The drawing under review shows one solid part. Ordinate dimensions are in mm from its lowest x, y, z. Give positions to 0.01 mm unless a question says otherwise; leave off trailing zeros. Loops run counter-clockwise (first coordinate to the right, second up) from the corner with the lowest first, then second, coordinate; pieces in that order, holes last. Notation, with made-up numbers: M 48,50 L 97,50 A13 cw 97,73 Z; hole C -35,24 d1. An arc over 180 degrees is marked long. One line per item, written item: value. Start each with the question number.
Q1. We need section C-C on y = 0.5. Write out the cut boundary in (x, z), plus the area to 3 significant figures.
Q2. For pin 1 (1.5 mm diameter, centred on y = 1, z = 1.5, fed in from -X), flat-tipped, find the tip position at first contact; note if it passes through.
Q3. We need section B-B on z = 2.4. Write out the cut boundary in (x, y).
Q4. We need section A-A on x = 19. Write out the cut boundary in (y, z), plus the area to 3 significant figures.
Q5. To check wall thickness, follow line 1 along Y through (x, z) = (6, 2.05); line 2 along Z through (x, y) = (20, 1.05); line 3 along Z through (x, y) = (12, 0.25). State the ranges of each line that lie inside material, in increasing order. Write a range as from..to.
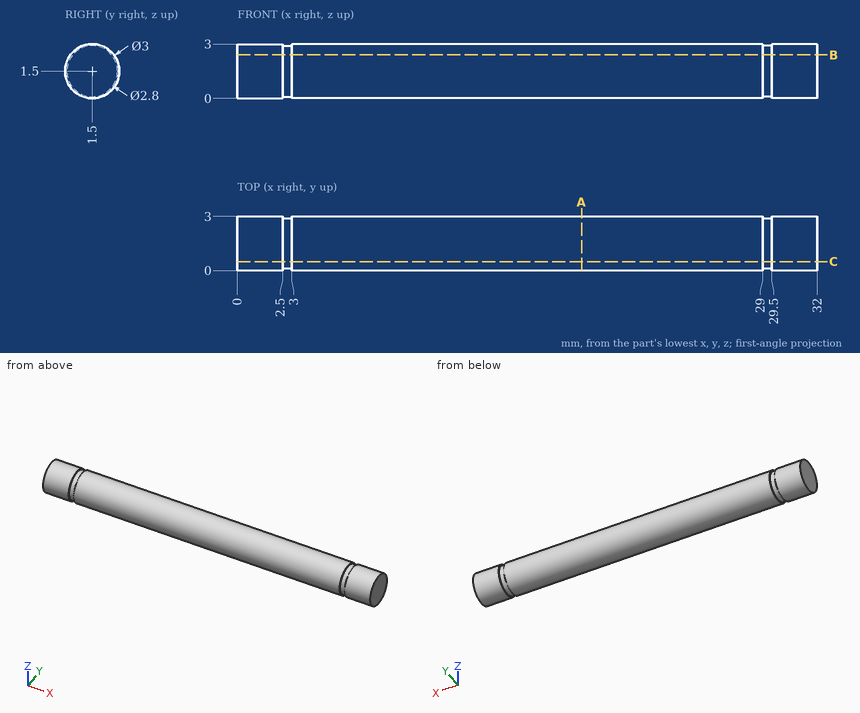
Solved:
1. outline: M 0,0.38 L 2.5,0.38 L 2.5,0.52 L 3,0.52 L 3,0.38 L 29,0.38 L 29,0.52 L 29.5,0.52 L 29.5,0.38 L 32,0.38 L 32,2.62 L 29.5,2.62 L 29.5,2.48 L 29,2.48 L 29,2.62 L 3,2.62 L 3,2.48 L 2.5,2.48 L 2.5,2.62 L 0,2.62 Z
1. area: 71.3 mm2
2. pin 1: x = 0
3. outline: M 0,0.3 L 2.5,0.3 L 2.5,0.43 L 3,0.43 L 3,0.3 L 29,0.3 L 29,0.43 L 29.5,0.43 L 29.5,0.3 L 32,0.3 L 32,2.7 L 29.5,2.7 L 29.5,2.57 L 29,2.57 L 29,2.7 L 3,2.7 L 3,2.57 L 2.5,2.57 L 2.5,2.7 L 0,2.7 Z
4. outline: C 1.5,1.5 d3
4. area: 7.07 mm2
5. line 1: 0.1..2.9
5. line 2: 0.07..2.93
5. line 3: 0.67..2.33
